Autodesk Inventor part; units mm, degrees
ref_plane "YZ Plane" through (0, 0, 0) normal (1, 0, 0) x (0, 1, 0)
ref_plane "XZ Plane" through (0, 0, 0) normal (0, 1, 0) x (-1, 0, 0)
ref_plane "XY Plane" through (0, 0, 0) normal (0, 0, 1) x (1, 0, 0)
sketch "Sketch1" plane through (0, 0, 0) normal (0, 0, 1) x (1, 0, 0)
  circle A0 centre (-10, 0) radius 1.5
  circle A1 centre (10, 0) radius 1.5
  circle A2 centre (-10, -20) radius 1.5
  circle A3 centre (10, -20) radius 1.5
  line L0 (-15, 10) -> (15, 10)
  line L1 (15, 10) -> (15, -30)
  line L2 (15, -30) -> (-15, -30)
  line L3 (-15, -30) -> (-15, 10)
  point P0 (0, 0)
  dimension "d0" = 3
  dimension "d1" = 3
  dimension "d2" = 20
  dimension "d3" = 10
  dimension "d4" = 3
  dimension "d5" = 3
  dimension "d6" = 20
  dimension "d7" = 20
  dimension "d8" = 20
  dimension "d9" = 10
  dimension "d10" = 30
  dimension "d11" = 15
  dimension "d12" = 40
  dimension "d13" = 10
extrude "Extrusion1" add sketch "Sketch1" along normal blind 5
sketch "Sketch2" plane through (0, 0, 5) normal (0, 0, 1) x (1, 0, 0)
  line L0 (0, 15.442053) -> (0, -37.541934) construction
  line L1 (-4, 15.442053) -> (-4, -37.541934) construction
  line L2 (-15, -30) -> (15, -30) construction
  line L3 (15, 10) -> (-15, 10)
  line L4 (15, -30) -> (15, 10)
  line L5 (7, 10) -> (7, -30)
  line L6 (7, 10) -> (15, 10)
  line L7 (7, -30) -> (15, -30)
  line L8 (6.3, 15.442053) -> (6.3, 10) construction
  line L9 (6.3, -30) -> (6.3, -37.541934) construction
  line L10 (-15, 10) -> (-15, -30)
  line L11 (15, -30) -> (15, 10)
  point P0 (0, 0)
  dimension "d16" = 4
  dimension "d96" = 0
  dimension "d97" = 0
  dimension "d141" = 22
  dimension "d152" = 0
extrude "Extrusion2" add sketch "Sketch2" along normal blind 10
sketch "Sketch4" plane through (0, 0, 15) normal (0, 0, 1) x (1, 0, 0)
  circle A0 centre (10, 0) radius 3.25
  circle A1 centre (10, -20) radius 1.5
  circle A2 centre (10, -20) radius 3.25
  point P0 (0, 0)
  point P1 (8.5, 0)
  point P2 (8.5, -20)
  dimension "d37" = 6.5
  dimension "d38" = 6.5
extrude "Extrusion3" [suppressed]
sketch "Sketch5" plane through (0, 0, 5) normal (0, 0, 1) x (1, 0, 0)
  line L0 (-4, 15.442053) -> (-4, -37.541934) construction
  line L1 (15, -30) -> (-15, -30)
  line L2 (7, 10) -> (-15, 10)
  line L3 (-3.3, 10) -> (1, 10)
  line L4 (4.5, -30) -> (-3.3, -30)
  line L5 (-3.3, -30) -> (-3.3, 10)
  line L6 (-2, 6) -> (1, 6)
  line L7 (4.5, -26) -> (-2, -26)
  line L8 (-2, -26) -> (-2, 6)
  line L9 (1, 10) -> (1, 6)
  line L10 (4.5, -26) -> (4.5, -30)
  line L11 (7, 10) -> (7, -30)
  point P0 (0, 0)
  point P1 (6.3, 10)
  point P2 (6.3, -30)
  point P3 (15, 10)
  dimension "d111" = 0.7
  dimension "d112" = 4
  dimension "d115" = 4
  dimension "d116" = 1.3
  dimension "d117" = 6
  dimension "d118" = 2.5
  dimension "d139" = 0
  dimension "d140" = 0
extrude "Extrusion4" add sketch "Sketch5" along normal up to surface (10 mm away) contours L1 L5 L2 L9 L6 L8 L7 L10
sketch "Sketch8" plane through (0, 0, 0) normal (0, 0, -1) x (-1, 0, 0)
  line L0 (27, -15) -> (-27, -15)
  line L1 (-27, -15) -> (-27, -5)
  line L2 (-27, -5) -> (27, -5)
  line L3 (27, -5) -> (27, -15)
  line L4 (15, 10) -> (-15, 10)
  line L5 (-15, -30) -> (15, -30)
  circle A0 centre (23, -10) radius 1.5
  circle A1 centre (-23, -10) radius 1.5
  point P0 (0, 0)
  dimension "d77" = 10
  dimension "d78" = 40
  dimension "d79" = 15
  dimension "d80" = 3
  dimension "d81" = 3
  dimension "d82" = 46
  dimension "d83" = 54
  dimension "d84" = 23
  dimension "d85" = 27
extrude "Extrusion5" add sketch "Sketch8" against normal up to surface (5 mm away)
sketch "Sketch3" plane through (0, 0, 5) normal (0, 0, 1) x (1, 0, 0)
  circle A0 centre (2, -2) radius 1.25
  circle A1 centre (2, -15) radius 1.25
  line L0 (-15, -30) -> (15, -30)
  line L1 (15, 10) -> (-15, 10)
  point P0 (0, 0)
  point P1 (7, -30)
  point P2 (6.3, 10)
  dimension "d23" = 2.5
  dimension "d24" = 2.5
  dimension "d25" = 15
  dimension "d26" = 2
  dimension "d27" = 2
  dimension "d28" = 12
hole "Hole1" at (2, -2, 5) at (2, -15, 5) direction (0, 0, -1) diameter 2.5 end through all
fillet "Fillet5" [suppressed]
fillet "Fillet7" [suppressed]
sketch "Sketch11" plane through (0, 0, 0) normal (0, 0, -1) x (-1, 0, 0)
  line L0 (15, -15) -> (13.5, -15)
  line L1 (13.5, -5) -> (15, -5)
  line L2 (-15, -5) -> (-13.5, -5)
  line L3 (-13.5, -15) -> (-15, -15)
  line L4 (15, -30) -> (15, -15)
  line L5 (-15, -15) -> (-15, -30)
  line L6 (-15, 10) -> (-15, -5)
  line L7 (15, -5) -> (15, 10)
  line L8 (-15, -30) -> (-13.5, -30)
  line L9 (13.5, -30) -> (15, -30)
  line L10 (-13.5, -30) -> (-13.5, -15)
  line L11 (-13.5, -5) -> (-13.5, 10)
  line L12 (13.5, 10) -> (13.5, -5)
  line L13 (13.5, -15) -> (13.5, -30)
  line L14 (15, 10) -> (13.5, 10)
  line L15 (-15, 10) -> (15, 10)
  line L16 (-15, 10) -> (-13.5, 10)
  point P0 (0, 0)
  dimension "d121" = 27
extrude "Extrusion7" cut sketch "Sketch11" against normal through all
fillet "Fillet9" radius 3 12 edges at (-27, -15, 2.5) (-13.5, -30, 2.5) (13.5, -30, 7.5) (-27, -5, 2.5) (-13.5, -5, 2.5) (-13.5, 10, 2.5) (13.5, -15, 7.5) (27, -15, 2.5) (27, -5, 2.5) (13.5, -5, 7.5) (13.5, 10, 7.5) (-13.5, -15, 2.5)
sketch "Sketch12" plane through (4, -30, 4) normal (0, -1, 0) x (1, 0, 0)
  line L0 (0.5, 11) -> (-7.3, 11)
  circle A0 centre (-2, 3) radius 1.5
  line L1 (0.5, 1) -> (3, 1)
  line L2 (6.5, -4) -> (-14.5, -4)
  line L3 (6.5, 11) -> (6.5, -4)
  line L4 (-14.5, -4) -> (-14.5, 1)
  line L5 (-7.3, 1) -> (-7.3, 11)
  line L6 (-14.5, 1) -> (-7.3, 1)
  line L7 (3, 11) -> (6.5, 11)
  line L8 (3, 1) -> (3, 11)
  line L9 (0.5, 1) -> (0.5, 11)
  point P0 (-4, -4)
  dimension "d126" = 3
  dimension "d129" = 3
extrude "Extrusion8" [suppressed]
sketch "Sketch14" plane through (0, 0, 0) normal (0, 0, -1) x (-1, 0, 0)
  line L0 (10.5, 10) -> (-10.5, 10)
  line L1 (-1, 10) -> (1, 10)
  line L2 (1, 10) -> (1, 24)
  line L3 (1, 24) -> (-1, 24)
  line L4 (-1, 24) -> (-1, 10)
  point P0 (0, 0)
  dimension "d142" = 14
  dimension "d143" = 1
  dimension "d144" = 1
extrude "Extrusion10" add sketch "Sketch14" against normal up to surface (15 mm away)
fillet "Fillet10" radius 3 2 edges at (-1, 10, 7.5) (1, 10, 2.5)
fillet "Fillet11" radius 1 2 edges at (-1, 24, 7.5) (1, 24, 7.5)
sketch "Sketch15" plane through (-3.3, -30, 15) normal (0, 0, 1) x (1, 0, 0)
  arc A0 (2.3, 53) -> (4.3, 53) centre (3.3, 53) ccw
  line L0 (2.3, 43) -> (2.3, 53)
  arc A1 (0, 40.08281) -> (2.3, 43) centre (-0.7, 43) ccw
  line L1 (0, 0) -> (0, 36)
  line L2 (7.8, 0) -> (0, 0)
  line L3 (7.8, 4) -> (7.8, 0)
  line L4 (1.3, 4) -> (7.8, 4)
  line L5 (1.3, 36) -> (1.3, 4)
  line L6 (4.3, 36) -> (1.3, 36)
  line L7 (4.3, 53) -> (4.3, 36)
  line L8 (7.3, 40) -> (7.8, 40)
  arc A2 (4.3, 43) -> (6.8, 40.04196) centre (7.3, 43) ccw
  line L9 (4.3, 53) -> (4.3, 36)
  line L10 (1.3, 36) -> (1.3, 4)
  line L11 (1.3, 36) -> (0, 36)
  line L12 (0, 0) -> (0, 36)
  point P0 (3.3, 30)
extrude "Extrusion11" cut sketch "Sketch15" against normal up to surface (10 mm away)
sketch "Sketch16" plane through (10, 0, 5) normal (0, 0, -1) x (-1, 0, 0)
  circle A0 centre (0, 0) radius 1.5
  circle A1 centre (0, -20) radius 1.5
  point P0 (10, 0)
extrude "Extrusion12" cut sketch "Sketch16" against normal through all
sketch "Sketch17" plane through (-3.3, 6, 15) normal (0, 0, 1) x (1, 0, 0)
  line L0 (4.3, 0) -> (0, 0)
  line L1 (4.3, 17) -> (4.3, 0)
  arc A0 (4.3, 17) -> (2.3, 17) centre (3.3, 17) ccw
  line L2 (2.3, 7) -> (2.3, 17)
  arc A1 (0, 4.08281) -> (2.3, 7) centre (-0.7, 7) ccw
  line L3 (0, 0) -> (0, 4.08281)
  point P0 (3.3, -6)
sketch "Sketch17 outline for Extrusion13" plane through (-3.3, 6, 15) normal (0, 0, 1) x (1, 0, 0)
  line L0 (0, 4.08281) -> (0, 0)
  arc A0 (2.3, 7) -> (0, 4.08281) centre (-0.7, 7) cw
  line L1 (2.3, 17) -> (2.3, 7)
  arc A1 (4.3, 17) -> (2.3, 17) centre (3.3, 17) ccw
  line L2 (4.3, 0) -> (4.3, 17)
  line L3 (0, 0) -> (4.3, 0)
extrude "Extrusion13" cut sketch "Sketch17 outline for Extrusion13" against normal up to surface (10 mm away)
sketch "Sketch18" plane through (0, 0, 15) normal (0, 0, 1) x (1, 0, 0)
  circle A0 centre (10, 0) radius 1.5
  circle A1 centre (10, -20) radius 1.5
  arc A2 (13.5, 7) -> (10.5, 10) centre (10.5, 7) ccw
  line L0 (10.5, 10) -> (7, 10)
  line L1 (7, 10) -> (7, -30)
  line L2 (7, -30) -> (10.5, -30)
  arc A3 (10.5, -30) -> (13.5, -27) centre (10.5, -27) ccw
  line L3 (13.5, -27) -> (13.5, -18)
  arc A4 (15, -15.401924) -> (13.5, -18) centre (16.5, -18) ccw
  line L4 (15, -4.598076) -> (15, -15.401924)
  arc A5 (13.5, -2) -> (15, -4.598076) centre (16.5, -2) ccw
  line L5 (13.5, -2) -> (13.5, 7)
  point P0 (0, 0)
extrude "Extrusion14" cut sketch "Sketch18" against normal up to surface (10 mm away)
sketch "Sketch13" plane through (-10.5, -30, 0) normal (0, -1, 0) x (1, 0, 0)
  line L0 (21, 4) -> (21, 0)
  line L1 (0, 0) -> (0, 4)
  line L2 (21, 0) -> (0, 0)
  circle A0 centre (11, 8) radius 1.5
  line L3 (19.5, 4) -> (21, 4)
  line L4 (19.5, 4) -> (19.5, 14)
  line L5 (17.5, 14) -> (19.5, 14)
  line L6 (17.5, 4) -> (17.5, 14)
  line L7 (15, 4) -> (17.5, 4)
  line L8 (15, 4) -> (15, 14)
  line L9 (15, 14) -> (7.2, 14)
  line L10 (7.2, 4) -> (7.2, 14)
  line L11 (0, 4) -> (7.2, 4)
  point P0 (10.5, 0)
  dimension "d132" = 3
  dimension "d133" = 21
  dimension "d134" = 4
  dimension "d136" = 11
  dimension "d149" = 8
sketch "Sketch9" plane through (0, 0, 5) normal (0, 0, 1) x (1, 0, 0)
  circle A0 centre (-10, 0) radius 1.5
  circle A1 centre (2, -2) radius 1.25
  circle A2 centre (10, 0) radius 1.5
  circle A3 centre (23, -10) radius 1.5
  circle A4 centre (10, -20) radius 1.5
  circle A5 centre (2, -15) radius 1.25
  circle A6 centre (-10, -20) radius 1.5
  circle A7 centre (-23, -10) radius 1.5
  point P0 (0, 0)
equation "\"d7\" = d6"
equation "\"d8\" = d2"
equation "\"d37\" = d38"
equation "\"d115\" = d112"
equation "\"d79\" = -0.5 * d77 + 0.5 * d78"
properties part number "vertical carriage vasi"
Work out the finished part from the listing and answer in its coordinate system (mm). A direction names the side the tool comes from. Give positions to 0.01 mm unless a question says otherwise; leave off trailing zeros. Order: outer loops, then holes, each group sorted by start corner. A loop starts at its lowest first (then second) coordinate and runs counter-clockwise, first axis right, second up.
1. Section A-A, the plane y = -10 is taken. Determine the outline of the cut face in (x, z), and give its area (3 significant figures).
Result sheet:
outline: (-27, 0) - (-24.5, 0) - (-24.5, 5) - (-27, 5) - close; (-21.5, 0) - (21.5, 0) - (21.5, 5) - (-21.5, 5) - close; (24.5, 0) - (27, 0) - (27, 5) - (24.5, 5) - close
area: 240 mm2
2. Each of these flat-tipped pins is pushed along its axis until it touches: P1, Ø1.5, axis at x = 8.5, z = 3.5, coming from the +Y side; P2, Ø2.5, axis at x = 23, y = -10, coming from the -Z side; P3, Ø2, axis at x = 20.5, z = 1.5, coming from the -Y side; P4, Ø8, axis at x = -3.5, y = 17, coming from the +Z side. Where does it stop, or does it pass through?
Result sheet:
P1: stops at y = 10
P2: passes through
P3: stops at y = -15
P4: stops at z = 5
3. Straight lines are drawn through the part: L1, parallel to Y at x = 10, z = 3.9; L2, parallel to Y at x = 2, z = 1.35; L3, parallel to X at y = 14, z = 3.4. For each, find the intervals that lie inside material, in ascending order.
Result sheet:
L1: y = -30 to -21.5, -18.5 to -1.5, 1.5 to 10
L2: y = -30 to -16.25, -13.75 to -3.25, -0.75 to 10.76
L3: x = -1 to 1
4. Section B-B, the plane x = 2 is taken. Determine the outline of the cut face in (y, z), and give its area (3 significant figures).
Result sheet:
outline: (-30, 0) - (-16.25, 0) - (-16.25, 5) - (-30, 5) - close; (-13.75, 0) - (-3.25, 0) - (-3.25, 5) - (-13.75, 5) - close; (-0.75, 0) - (10.76, 0) - (10.76, 5) - (-0.75, 5) - close
area: 179 mm2
5. Section D-D, the plane x = 17.5 is taken. Determine the outline of the cut face in (y, z).
Result sheet:
outline: (-15, 0) - (-5, 0) - (-5, 5) - (-15, 5) - close
6. The mould has two halves that part along Y. Classify faces 1 (the cylindrical face through (8.5, -0.07, 2.46)), 2 (the cylindrical face through (-12.64, 9.1, 2.46)), 3 (the flat face through (0, -9, 0)): released by +Y, released by -Y, zero draft, split by the parting line, or undercut.
Result sheet:
face 1: undercut
face 2: released by +Y
face 3: zero draft
7. Section C-C, the plane z = 4 is taken. Give the number of separate pieces and of enclosed holes in the cut face, and give its area (3 significant figures).
Result sheet:
separate pieces: 1
enclosed holes: 8
area: 1,320 mm2
8. For faces 4 (the flat face through (1, 18, 2)), 5 (the flat face through (0, -9, 5)), determine the directions among +Z, -Z, +X, -X, +Y, -Y from which every point of the face is accessible in a straight line to the end or side of a thin tool.
Result sheet:
face 4: +Z, -Z, +X, +Y
face 5: +Z, +X, -X, +Y, -Y
